```python
from build123d import *

# Parameters (mm, degrees)
F0_W     = 27.94
F0_H     = 33.02
F1_DEPTH = 17.78
F2_T     = -2.54
F3_R     = 2.54
F5_D     = 7.62
F7_D     = 7.62
F9_D     = 2.54
F11_D    = 2.54


# Not quite as in the source:
# - a feature names something its author has since deleted; it is built from what else it names


with BuildPart() as f1:
    # F0 (on Front) → F1 (new body, symmetric)
    with BuildSketch(Plane.XZ):
        Rectangle(F0_W, F0_H)
    extrude(amount=F1_DEPTH, both=True)

    # F2
    f2_openings = [f1.faces().sort_by_distance(p)[0] for p in [
        (0, 0, 16.51),
        (-13.97, 0, 0),
        (13.97, 0, 0),
    ]]
    offset(amount=F2_T, openings=f2_openings)

    # F3
    f3_edges = [f1.edges().sort_by_distance(p)[0] for p in [
        (0, 17.78, -16.51),
        (0, -17.78, -16.51),
    ]]
    fillet(f3_edges, radius=F3_R)

    # F5 (through all)
    with Locations(Plane.XY.offset(-13.97)):
        with Locations((0, 0)):
            Hole(F5_D / 2)

    # F7 (through all)
    with Locations(Plane(origin=(0, 17.78, 0), x_dir=(-1, 0, 0), z_dir=(0, 1, 0))):
        with Locations((0, 1.2737165671)):
            Hole(F7_D / 2)

    # F9 (through all)
    with Locations(Plane.XZ.offset(17.78)):
        with Locations((-5.4043098353, 6.6219973378), (0, 8.9699165671), (5.6151403114, 6.673975382), (7.6956628408, 1.2737165671), (5.7190973312, -4.3454747647), (0, -6.4224834329), (-5.6642023847, -3.8776681758), (-7.6962, 1.2737165671)):
            Hole(F9_D / 2)

    # F11 (through all)
    with Locations(Plane(origin=(0, 0, -16.51), x_dir=(1, 0, 0), z_dir=(0, 0, -1))):
        with Locations((-5.1595509827, 5.7105628529), (0, 7.6962), (5.2015446278, 5.6723388408), (7.6962, 0), (-5.7603712318, -5.1038826115), (-7.6962, 0), (0, -7.6962), (5.5570431587, -5.3245437149)):
            Hole(F11_D / 2)


solid = f1.part
```
The listing builds one solid part. Answer for the finished solid, in the listing's coordinates (mm). A direction names the side the tool comes from. Coordinates: 2 decimals unless noted, no trailing zeros. Loops run counter-clockwise (first coordinate to the right, second up) from the corner with the lowest first, then second, coordinate; pieces in that order, holes last. Notation, with made-up numbers: (-32, 3) -> (19, 3) arc R16 cw to (19, 18) -> close; hole circle Ø6 at (-16, 33). An arc over 180 degrees is marked (long way). Return JSON: item names as keys, results as strings. Group by question number.
(1) A cutting plane is placed at C-C on x = -5.25. Count the separate pieces of the cut face and the enclosed holes in it, and give its area (3 significant figures).
(2) Given pin 1 Ø4 at (x, y) = (-2.5, 8) entering from +Z, flat-ended and moving along its own axis, determine where the tip first touches the part or whether it passes through.
(3) Find the intervals of material crossed by probe 1 along Y at (x, z) = (-8.5, 7); probe 2 along Y at (x, z) = (0, -15.2); probe 3 along Z at (x, y) = (0, -16.2), in increasing order. Write a range as from..to.
(4) A cutting plane is placed at B-B on y = 0. Write down the section's boundary in (x, z), and give its area (3 significant figures).
(5) Determine the mould class of faces 1 (the flat face through (0, -17, 16.51)), 2 (the flat face through (-3, 17.78, 5)), 3 (the cylindrical face through (0.275, -6.456, -15.222)), 4 (the cylindrical face through (0.165, 6.437, -15.222)) for opening direction Y: released by +Y, released by -Y, zero draft, split by the parting line, or undercut.
(6) Which of the six approach directions +Z, -Z, +X, -X, +Y, -Y give full straight-line access (tool end or side, diameter ignored) to faces 5 (the cylindrical face through (-4.49, 5.05, -15.22)), 6 (the flat face through (-3, -4, -13.97))?
(7) A cutting plane is placed at A-A on z = -10. Write down the section's boundary in (x, y).
The answers:
{
 "1": {"separate pieces": "7", "enclosed holes": "0", "area": "205 mm^2"},
 "2": {"pin 1": "stops at z = -13.97"},
 "3": {"probe 1": "y = -17.78..-15.24, 15.24..17.78", "probe 2": "y = -17.46..-8.97, -6.43..-3.81, 3.81..6.43, 8.97..17.46", "probe 3": "z = -16.32..-7.69, -5.15..-2.54, 5.08..7.7, 10.24..16.51"},
 "4": {"outline": "(-13.97, -16.51) -> (-8.97, -16.51) -> (-8.97, -13.97) -> (-13.97, -13.97) -> close; (-6.43, -16.51) -> (-3.81, -16.51) -> (-3.81, -13.97) -> (-6.43, -13.97) -> close; (3.81, -16.51) -> (6.43, -16.51) -> (6.43, -13.97) -> (3.81, -13.97) -> close; (8.97, -16.51) -> (13.97, -16.51) -> (13.97, -13.97) -> (8.97, -13.97) -> close", "area": "38.7 mm^2"},
 "5": {"face 1": "zero draft", "face 2": "released by +Y", "face 3": "undercut", "face 4": "undercut"},
 "6": {"face 5": "+Z, -Z", "face 6": "+Z, +X, -X"},
 "7": {"outline": "(-13.97, -17.78) -> (13.97, -17.78) -> (13.97, -15.24) -> (-13.97, -15.24) -> close; (-13.97, 15.24) -> (13.97, 15.24) -> (13.97, 17.78) -> (-13.97, 17.78) -> close"}
}
